CAD build for the part. Positions are in the model's coordinates, mm. A direction names the side the tool comes from. Coordinates: 2 decimals unless noted, no trailing zeros. Order: outer loops, then holes, each group sorted by start corner. A loop starts at its lowest first (then second) coordinate and runs counter-clockwise, first axis right, second up. Notation, with made-up numbers: (18, 14.5) - (47, 14.5) arc R9 cw to (47, 25.5) - close; hole circle Ø4 at (62, 60.25). An arc over 180 degrees is marked (long way). Use one line per item in the form item = value.
```python
from build123d import *

# Parameters (mm, degrees)
F0_W     = 25.4
F0_H     = 25.4
F0_W_2   = 22.225
F0_H_2   = 22.225
F1_DEPTH = 304.8
F2_R     = 3.175
F3_DEPTH = 1.5875
F4_R     = 2.15265
F5_DEPTH = 25.4
F6_R     = 4.7625
F7_DEPTH = 1.5875
F8_R     = 4.7625
F9_DEPTH = 1.5875


with BuildPart() as f1:
    # F0 (on Top) → F1 (new body)
    with BuildSketch(Plane.XY):
        Rectangle(F0_W, F0_H)
        Rectangle(F0_W_2, F0_H_2, mode=Mode.SUBTRACT)
    extrude(amount=F1_DEPTH)

    # F2 (on face) → F3 (cut, through all)
    with BuildSketch(Plane(origin=(0, 12.7, 0), x_dir=(-1, 0, 0), z_dir=(0, 1, 0))):
        with Locations((0, 152.4)):
            Circle(F2_R)
    extrude(amount=-F3_DEPTH, mode=Mode.SUBTRACT)

    # F4 (on face) → F5 (cut, through all)
    with BuildSketch(Plane(origin=(-12.7, 0, 0), x_dir=(0, -1, 0), z_dir=(-1, 0, 0))):
        with Locations((0, 12.7)):
            Circle(F4_R)
        with Locations((0, 165.1)):
            Circle(F4_R)
        with Locations((0, 292.1)):
            Circle(F4_R)
        with Locations((0, 215.9)):
            Circle(F4_R)
    extrude(amount=-F5_DEPTH, mode=Mode.SUBTRACT)

    # F6 (on face) → F7 (cut, through all)
    with BuildSketch(Plane.YZ.offset(12.7)):
        with Locations((0, 292.1)):
            Circle(F6_R)
        with Locations((0, 215.9)):
            Circle(F6_R)
    extrude(amount=-F7_DEPTH, mode=Mode.SUBTRACT)

    # F8 (on face) → F9 (cut, through all)
    with BuildSketch(Plane(origin=(-12.7, 0, 0), x_dir=(0, -1, 0), z_dir=(-1, 0, 0))):
        with Locations((0, 165.1)):
            Circle(F8_R)
        with Locations((0, 12.7)):
            Circle(F8_R)
    extrude(amount=-F9_DEPTH, mode=Mode.SUBTRACT)


solid = f1.part
```
Item 1: Cut at B-B, the plane z = 152.4. Write the cut outline in (x, y) (1 decimal).
Derived:
outline = (-12.7, -12.7) - (12.7, -12.7) - (12.7, 12.7) - (3.2, 12.7) - (3.2, 11.1) - (11.1, 11.1) - (11.1, -11.1) - (-11.1, -11.1) - (-11.1, 11.1) - (-3.2, 11.1) - (-3.2, 12.7) - (-12.7, 12.7) - close
Item 2: 3-axis set-ups, long thin cutter, end or side, ignore diameter. For faces 5 (the face through (-11.3, 0.1, 304.8)), 6 (the face through (0.41, 11.92, 155.55)), 7 (the face through (-11.92, 1.03, 8.05)), 8 (the face through (-12.7, 0, 150)), 9 (the face through (-11.112, 0, 150)): which of +Z, -Z, +X, -X, +Y, -Y reach the whole face in a straight line?
Derived:
face_5 = +Z, +X, -X, +Y, -Y
face_6 = +Y
face_7 = -X
face_8 = +Z, -Z, -X, +Y, -Y
face_9 = +Z, -Z
Item 3: Drop flat-ended pins along their axis: pin 1 (12.5 mm diameter, centred on y = 0, z = 165.1, fed in from +X); pin 2 (5.5 mm diameter, centred on y = 0, z = 215.9, fed in from +X); pin 3 (5.5 mm diameter, centred on x = 0, z = 152.4, fed in from +Y). Give the stop position or say it passes through.
Derived:
pin_1 = 12.7
pin_2 = -11.11
pin_3 = -11.11
Item 4: Drill centre lines: line 1 (Z direction, x = -11.45, y = 0); line 2 (Z direction, x = 0, y = 11.6) (3 decimals); line 3 (X direction, y = -2.25, z = 56.5). Where is each one in solid material? Low to high. Write a range as [from, to].
Derived:
line_1 = [0, 7.94], [17.46, 160.34], [169.86, 213.75], [218.05, 289.95], [294.25, 304.8]
line_2 = [0, 149.225], [155.575, 304.8]
line_3 = [-12.7, -11.11], [11.11, 12.7]
Item 5: Cut at C-C, the plane z = 204.5. Write the cut outline in (x, y), plus the area to 3 significant figures.
Derived:
outline = (-12.7, -12.7) - (12.7, -12.7) - (12.7, 12.7) - (-12.7, 12.7) - close; hole (-11.11, -11.11) - (11.11, -11.11) - (11.11, 11.11) - (-11.11, 11.11) - close
area = 151 mm²
Item 6: Cut at A-A, the plane x = -7.75. Write the cut outline in (y, z).
Derived:
outline = (-12.7, 0) - (-11.11, 0) - (-11.11, 304.8) - (-12.7, 304.8) - close; (11.11, 0) - (12.7, 0) - (12.7, 304.8) - (11.11, 304.8) - close
Item 7: Two-plate mould, pull along Z, no slides. Class faces 1 (the face through (11.92, -1.03, 287.45)), 2 (the face through (-11.3, 0.1, 0)), 3 (the face through (3, 12.7, 150)), 4 (the face through (11.92, -0.62, 220.62)): +Z half, -Z half, draft (parallel to the pull), parting line (faces both ways), or undercut.
Derived:
face_1 = undercut
face_2 = -Z half
face_3 = draft
face_4 = undercut
